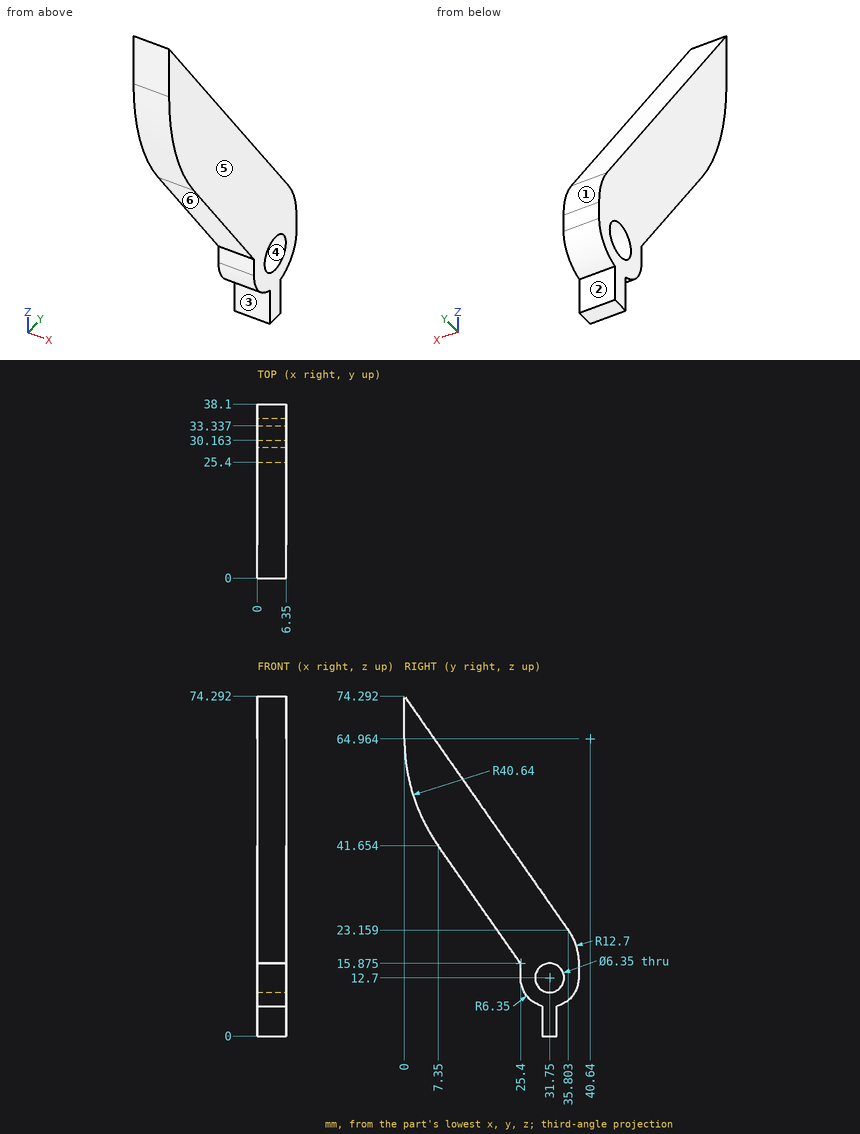
Geometry: see drawing. Coordinates: mm, zero at the bounding-box minimum. A direction names the side the tool comes from. Give positions to 0.01 mm unless a question says otherwise; leave off trailing zeros. Answer in a Markdown table with one row per item. Add a question column.
(1) First-contact query: pin 1 (3.5 mm diameter, centred on x = 2.5, z = 14.5, fed in from -Y); pin 2 (10 mm diameter, centred on y = 31.75, z = 12.7, fed in from +X); pin 3 (1 mm diameter, centred on x = 1.5, z = 13.5, fed in from -Y); pin 4 (3 mm diameter, centred on x = 3.5, z = 52, fed in from -Y). Flat tips, straight axial feed; report the tip coordinate or a pass-through.
(2) Mould query, pull axis Z, two halves, no side actions, for the marked faces 4, 5 and 6. Classes: +Z half, -Z half, draft (parallel to the pull), parting line (faces both ways), or undercut.
(3) Ray query, line 1 (Y direction, x = 3.5, z = 12.7) (1 decimal); line 2 (Z direction, x = 3.5, y = 13) (1 decimal); line 3 (Y direction, x = 1, z = 14.5) (1 decimal). Return the intervals inside material, ascending.
(4) Reachability of the marked faces 1, 2 and 3 from +Z, -Z, +X, -X, +Y, -Y: full face, straight path, thin tool, end or side. Return the list, or none.
Result set:
| question | item | result |
|---|---|---|
| 1 | pin 1 | stops at y = 25.14 |
| 1 | pin 2 | stops at x = 6.35 |
| 1 | pin 3 | stops at y = 25.4 |
| 1 | pin 4 | stops at y = 1.65 |
| 2 | face 4 | undercut |
| 2 | face 5 | draft |
| 2 | face 6 | -Z half |
| 3 | line 1 | y = 25.4 to 28.6, 34.9 to 38.1 |
| 3 | line 2 | z = 33.6 to 55.7 |
| 3 | line 3 | y = 25.4 to 29.1, 34.4 to 38.1 |
| 4 | face 1 | +Z, +X, -X, +Y |
| 4 | face 2 | -Z, +X, -X, +Y |
| 4 | face 3 | -Z, +X, -X, -Y |
